CAD build for the part. Positions are in the model's coordinates, mm. A direction names the side the tool comes from. Give positions to 0.01 mm unless a question says otherwise; leave off trailing zeros. Write each loop counter-clockwise with the first axis right and the second up, starting at its lowest first coordinate (ties: lowest second). Pieces come first, ordered by that corner, then holes. Notation, with made-up numbers: (68.25, 78.25) -> (75.25, 78.25) arc R24 cw to (75.25, 109.25) -> close; hole circle Ø9 at (71, 83.5). An arc over 180 degrees is marked (long way). Answer as a JSON object with one key per item and string values.
```python
from build123d import *

# Parameters (mm, degrees)
SKETCH_1_R          = 20.5
EXTRUDE_1_DEPTH     = 50
FILLET_1_R          = 1
FILLET_2_R          = 1
SKETCH_2_R          = 2
CUT_EXTRUDE_1_DEPTH = 68.832514358
CUT_EXTRUDE_2_DEPTH = 2.4


with BuildPart() as part:
    # Эскиз1 → Бобышка-Вытянуть1 (new body)
    with BuildSketch(Plane.XY):
        Circle(SKETCH_1_R)
    extrude(amount=EXTRUDE_1_DEPTH)

    # Скругление1
    fillet_1_edges = [part.edges().sort_by_distance(p)[0] for p in [
        (-20.5, 0, 50),
    ]]
    fillet(fillet_1_edges, radius=FILLET_1_R)

    # Скругление2
    fillet_2_edges = [part.edges().sort_by_distance(p)[0] for p in [
        (-20.5, 0, 0),
    ]]
    fillet(fillet_2_edges, radius=FILLET_2_R)

    # Эскиз2 → Вырез-Вытянуть1 (cut, through all)
    with BuildSketch(Plane(origin=(20.5, 0, 0), x_dir=(0, 0, -1), z_dir=(1, 0, 0))):
        with Locations((-37.5, 0)):
            Circle(SKETCH_2_R)
        with Locations((-25, 0)):
            Circle(SKETCH_2_R)
        with Locations((-12.5, 0)):
            Circle(SKETCH_2_R)
    extrude(amount=-CUT_EXTRUDE_1_DEPTH, mode=Mode.SUBTRACT)

    # Эскиз3 → Вырез-Вытянуть2 (cut)
    with BuildSketch(Plane(origin=(20.5, 0, 0), x_dir=(0, 0, -1), z_dir=(1, 0, 0))):
        Polygon((-25, 3.175426481), (-27.75, 1.58771324), (-27.75, -1.58771324), (-25, -3.175426481), (-22.25, -1.58771324), (-22.25, 1.58771324), align=None)
        Polygon((-37.5, 3.175426481), (-40.25, 1.58771324), (-40.25, -1.58771324), (-37.5, -3.175426481), (-34.75, -1.58771324), (-34.75, 1.58771324), align=None)
        Polygon((-12.5, 3.175426481), (-15.25, 1.58771324), (-15.25, -1.58771324), (-12.5, -3.175426481), (-9.75, -1.58771324), (-9.75, 1.58771324), align=None)
    cut_extrude_2 = extrude(amount=-CUT_EXTRUDE_2_DEPTH, mode=Mode.SUBTRACT)

    # Зеркальное отражение1: Вырез-Вытянуть2 across plane
    add(cut_extrude_2.mirror(Plane(origin=(0, 0, 0), x_dir=(0, 0, 1), z_dir=(1, 0, 0))), mode=Mode.SUBTRACT)


solid = part.part
```
1) 3-axis set-ups, long thin cutter, end or side, ignore diameter. For faces 1 (the cylindrical face through (0.3, -1.2, 14.1)), 2 (the flat face through (19.29, 2.39, 13.86)), 3 (the flat face through (-19.29, -2.39, 23.64)): which of +Z, -Z, +X, -X, +Y, -Y reach the whole face in a straight line?
Model answer:
{"face 1": "+X, -X", "face 2": "+X", "face 3": "-X"}
2) Wall check: probe 1 along Y at (x, z) = (1, 12); probe 2 along Y at (x, z) = (7, 25); probe 3 along Y at (x, z) = (-7, 34.5). Give the ranges that are in metal, low to high.
Model answer:
{"probe 1": "y = -20.48 to -1.94, 1.94 to 20.48", "probe 2": "y = -19.27 to -2, 2 to 19.27", "probe 3": "y = -19.27 to 19.27"}
3) Slice it at A-A (x = 0). List the corners of the cut face in (y, z).
Model answer:
{"outline": "(-20.5, 1) arc R1 ccw to (-19.5, 0) -> (19.5, 0) arc R1 ccw to (20.5, 1) -> (20.5, 49) arc R1 ccw to (19.5, 50) -> (-19.5, 50) arc R1 ccw to (-20.5, 49) -> close; hole circle Ø4 at (0, 12.5); hole circle Ø4 at (0, 25); hole circle Ø4 at (0, 37.5)"}
4) Pin check, flat tips, straight feed: pin 1 (1 mm diameter, centred on x = 2.5, z = 13.5, fed in from -Y); pin 2 (3 mm diameter, centred on y = 0, z = 25, fed in from -X); pin 3 (1.5 mm diameter, centred on y = -14.5, z = 37, fed in from -X); pin 4 (10 mm diameter, centred on y = -11, z = 8.5, fed in from +X). Stop position of each tip, or through.
Model answer:
{"pin 1": "stops at y = -20.4", "pin 2": "passes through", "pin 3": "stops at x = -15.2", "pin 4": "stops at x = 19.6"}
5) Mould opens along Z. For faces 4 (the flat face through (19.286, -2.37, 13.894)), 5 (the flat face through (0, 0, 50)) say: released by +Z, released by -Z, zero draft, split by the parting line, or undercut.
Model answer:
{"face 4": "undercut", "face 5": "released by +Z"}
6) Slice it at B-B (y = 0). State how many separate pieces and enclosed holes the cut face has, then the cut area to 3 significant figures.
Model answer:
{"separate pieces": "4", "enclosed holes": "0", "area": "1,540 mm2"}
7) Slice it at C-C (z = 41.5). List the corners of the cut face in (x, y), then the cut area to 3 significant figures.
Model answer:
{"outline": "circle Ø41 at (0, 0)", "area": "1,320 mm2"}
